Work out the finished part from the listing and answer in its coordinate system (mm). A direction names the side the tool comes from. Round coordinates to 2 decimals unless told otherwise and drop trailing zeros. Loops run counter-clockwise (first coordinate to the right, second up) from the corner with the lowest first, then second, coordinate; pieces in that order, holes last. Notation, with made-up numbers: (-25, 54) - (-5, 54) arc R9 ccw to (-5, 59) - close; hole circle Ø9 at (6.5, 88). An arc over 180 degrees is marked (long way). Return JSON: item names as keys, results as strings.
from build123d import *

# Parameters (mm, degrees)
F0_R     = 45
F0_R_2   = 18.5
F1_DEPTH = 10
F2_R     = 42
F2_R_2   = 18.5
F3_DEPTH = 50
F5_DEPTH = 79.80825


with BuildPart() as f1:
    # F0 (on Top) → F1 (new body)
    with BuildSketch(Plane.XY):
        Circle(F0_R)
        Circle(F0_R_2, mode=Mode.SUBTRACT)
    extrude(amount=F1_DEPTH)

    # F2 (on face) → F3 (join)
    with BuildSketch(Plane.XY.offset(10)):
        Circle(F2_R)
        Circle(F2_R_2, mode=Mode.SUBTRACT)
    extrude(amount=F3_DEPTH)

    # F4 (on face) → F5 (cut)
    with BuildSketch(Plane.XY.offset(60)):
        Polygon((64.068409, 63.324335), (0, 63.324335), (0, 34.5), (5.733575, 34.5), (5.733575, 24.5), (0, 24.5), (0, -24.5), (-6.004329, -24.5), (-6.004329, -34.5), (0, -34.5), (0, -52.819867), (64.068409, -52.819867), align=None)
    extrude(amount=-F5_DEPTH, mode=Mode.SUBTRACT)


solid = f1.part
1) Section D-D (x = -30) is taken. Give the vertices of the cut face in (y, z), and give its area (3 significant figures).
Verdict:
{"outline": "(-33.54, 0) - (33.54, 0) - (33.54, 10) - (29.39, 10) - (29.39, 60) - (-29.39, 60) - (-29.39, 10) - (-33.54, 10) - close", "area": "3,610 mm2"}
2) Section B-B (z = 39) is taken. Give the vertices of the cut face in (x, y), and give its area (3 significant figures).
Verdict:
{"outline": "(-6, -34.5) - (-6, -24.5) - (0, -24.5) - (0, -18.5) arc R18.5 cw to (0, 18.5) - (0, 24.5) - (5.73, 24.5) - (5.73, 34.5) - (0, 34.5) - (0, 42) arc R42 ccw to (0, -42) - (0, -34.5) - close", "area": "2,230 mm2"}
3) Flat-ended cylindrical pins translate along their axes: pin 1 (1.8 mm diameter, centred on y = 21.5, z = 39, fed in from +X); pin 2 (4 mm diameter, centred on x = -2, z = 39.5, fed in from -Y); pin 3 (4.5 mm diameter, centred on x = 2.5, z = 39, fed in from +Y). Find the tip coordinate at first contact, or state that the pin passes through.
Verdict:
{"pin 1": "stops at x = 0", "pin 2": "stops at y = -42", "pin 3": "stops at y = 34.5"}
4) Section A-A (x = -7) is taken. Give the vertices of the cut face in (y, z), and give its area (3 significant figures).
Verdict:
{"outline": "(-44.45, 0) - (-17.12, 0) - (-17.12, 60) - (-41.41, 60) - (-41.41, 10) - (-44.45, 10) - close; (17.12, 0) - (44.45, 0) - (44.45, 10) - (41.41, 10) - (41.41, 60) - (17.12, 60) - close", "area": "2,980 mm2"}
5) A tool of negligible diameter and unlimited length cuts with its end or side. For faces 1 (the cylindrical face through (-41.99, 0.92, 34.65)), 2 (the flat face through (-3, -24.5, 30)), 3 (the cylindrical face through (-44.99, 0.99, 4.93)), 4 (the flat face through (0, -39, 30)), 5 (the flat face through (3, 34.5, 30)), from which of +Z, -Z, +X, -X, +Y, -Y can it reach the whole face along a straight path? Write none if from no direction.
Verdict:
{"face 1": "+Z, -X", "face 2": "+Z, -Z, +X", "face 3": "+Z, -Z, -X", "face 4": "+Z, -Z, +X, -Y", "face 5": "+Z, -Z, +X, +Y"}
6) Section C-C (y = 0) is taken. Give the vertices of the cut face in (x, z).
Verdict:
{"outline": "(-45, 0) - (-18.5, 0) - (-18.5, 60) - (-42, 60) - (-42, 10) - (-45, 10) - close"}
7) Find the intervals of material crossed by L1, parallel to Y at x = -3, z = 20.5; L2, parallel to Y at x = -3.5, z = 34.5; L3, parallel to Z at x = -35, y = 27, in increasing order.
Verdict:
{"L1": "y = -41.89 to -34.5, -24.5 to -18.26, 18.26 to 41.89", "L2": "y = -41.85 to -34.5, -24.5 to -18.17, 18.17 to 41.85", "L3": "z = 0 to 10"}
8) Determine the mould class of faces 6 (the flat face through (3, 24.5, 30)), 7 (the flat face through (0, 22, 30)), 8 (the flat face through (-6.004, -29, 30)) for opening direction Y: pulls with the +Y half, pulls with the -Y half, needs draft (parallel to the pull), parting line crosses it, or undercut.
Verdict:
{"face 6": "pulls with the -Y half", "face 7": "needs draft", "face 8": "undercut"}
